Verification items for this drawing (mm, ordinates from the low corner). Coordinates: 2 decimals unless noted, no trailing zeros. Order: outer loops, then holes, each group sorted by start corner. A loop starts at its lowest first (then second) coordinate and runs counter-clockwise, first axis right, second up. Notation, with made-up numbers: (50, -15.5) - (55, -15.5) arc R15 ccw to (55, 3.5) - close; hole circle Ø3 at (-8, 44). An arc over 180 degrees is marked (long way). Use CSV: the item, a comma, the result in double quotes. Start each with the question number.
1) Sectioned sample at B-B, the plane y = 0.7. Record the cut outline in (x, z).
2) Sectioned sample at C-C, the plane x = 4. Record the cut outline in (y, z), and give its area (3 significant figures).
3) Thickness scan on probe 1 along X at (y, z) = (2.55, 20); probe 2 along X at (y, z) = (4, 4); probe 3 along X at (y, z) = (3.5, 15.5) (3 decimals). Record the ranges inside material, lowest first. Write a range as [from, to].
4) Sectioned sample at D-D, the plane z = 26.5. Record the cut outline in (x, y) (3 decimals), and give its area (4 significant figures).
5) Sectioned sample at A-A, the plane z = 4. Record the cut outline in (x, y).
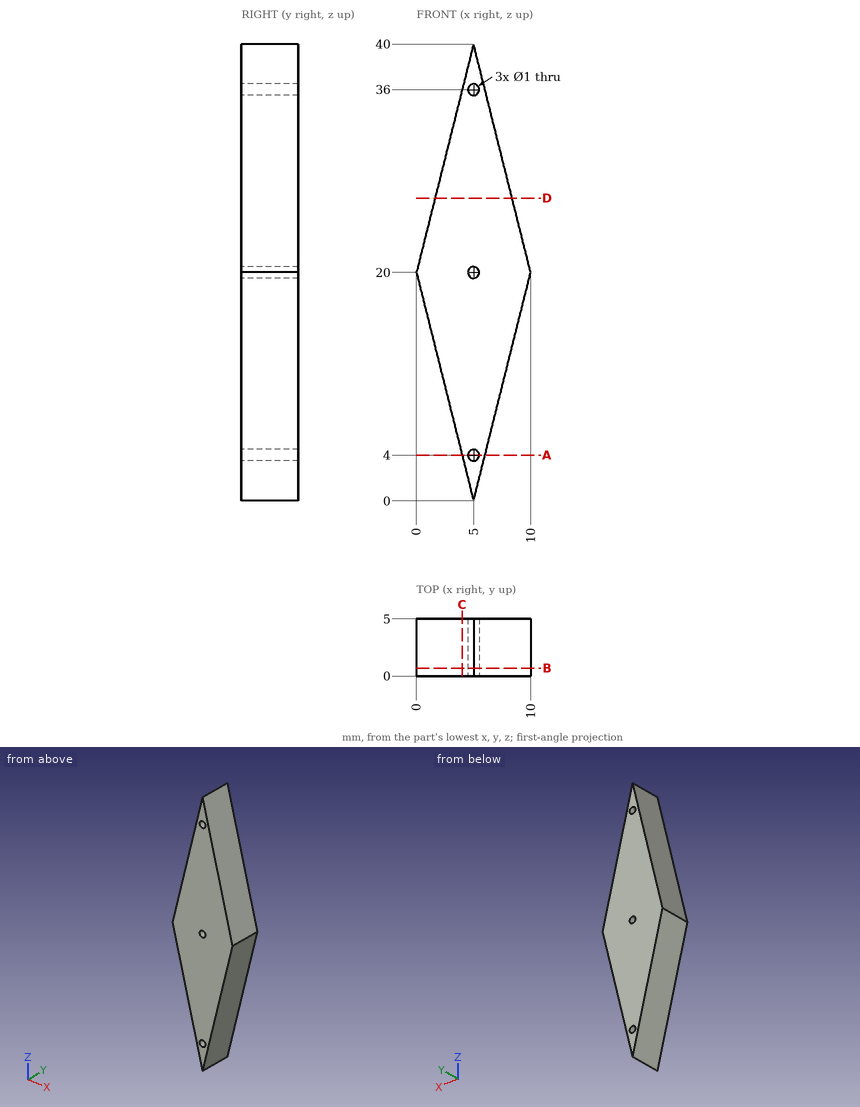
Evaluation:
1,outline,"(0, 20) - (5, 0) - (10, 20) - (5, 40) - close; hole circle Ø1 at (5, 4); hole circle Ø1 at (5, 20); hole circle Ø1 at (5, 36)"
2,outline,"(0, 4) - (5, 4) - (5, 36) - (0, 36) - close"
2,area,"160 mm²"
3,probe 1,"[0, 4.5], [5.5, 10]"
3,probe 2,"[4, 4.5], [5.5, 6]"
3,probe 3,"[1.125, 8.875]"
4,outline,"(1.625, 0) - (8.375, 0) - (8.375, 5) - (1.625, 5) - close"
4,area,"33.75 mm²"
5,outline,"(4, 0) - (4.5, 0) - (4.5, 5) - (4, 5) - close; (5.5, 0) - (6, 0) - (6, 5) - (5.5, 5) - close"
